Input: part model. Units: mm. Frame: model coordinates. A direction names the side the tool comes from. Round coordinates to 2 decimals unless told otherwise and drop trailing zeros. Loops run counter-clockwise (first coordinate to the right, second up) from the corner with the lowest first, then second, coordinate; pieces in that order, holes last. Notation, with made-up numbers: (-14.5, 50) - (5.5, 50) arc R18 ccw to (5.5, 59) - close; hole circle Ø2 at (-14.75, 70.5). An arc over 180 degrees is marked (long way). Write each question's results on one line, items separated by ' | '.
from build123d import *

# Parameters (mm, degrees)
SKETCH1_R               = 1.45
BOSS_EXTRUDE1_DEPTH     = 5
SKETCH2_R               = 1.45
BOSS_EXTRUDE2_DEPTH     = 2.6
SKETCH3_R               = 1.45
BOSS_EXTRUDE3_DEPTH     = 3
SKETCH5_W               = 3
SKETCH5_H               = 52.5
CHAMFER1_SIZE           = 1
SKETCH6_R               = 0.75
CUT_EXTRUDE1_DEPTH      = 5.0000001
CUT_EXTRUDE1_DEPTH_BACK = 5.0000001


with BuildPart() as part:
    # Sketch1 → Boss-Extrude1 (new body)
    with BuildSketch(Plane(origin=(0, 0, 0), x_dir=(0, 0, -1), z_dir=(1, 0, 0))):
        with BuildLine():
            Line((-4, 0), (-4, 6.5))
            ThreePointArc((-4, 6.5), (0, 10.5), (4, 6.5))
            Line((4, 6.5), (4, 0))
            ThreePointArc((4, 0), (0, -4), (-4, 0))
        make_face()
        with Locations((0, 6.5)):
            Circle(SKETCH1_R, mode=Mode.SUBTRACT)
    extrude(amount=BOSS_EXTRUDE1_DEPTH)

    # Sketch2 → Boss-Extrude2 (add)
    with BuildSketch(Plane(origin=(5, 0, 0), x_dir=(0, 0, -1), z_dir=(1, 0, 0))):
        with Locations((0, 0.05)):
            Circle(SKETCH2_R)
    extrude(amount=BOSS_EXTRUDE2_DEPTH)

    # Sketch3 → Boss-Extrude3 (add)
    with BuildSketch(Plane.ZY):
        with BuildLine():
            ThreePointArc((-4, 6.5), (0, 2.5), (4, 6.5))
            ThreePointArc((4, 6.5), (0, 10.5), (-4, 6.5))
        make_face()
        with Locations((0, 6.5)):
            Circle(SKETCH3_R, mode=Mode.SUBTRACT)
    extrude(amount=BOSS_EXTRUDE3_DEPTH)

    # Sketch5 → Revolve2 (revolve)
    with BuildSketch(Plane.XY):
        with Locations((2.5, 34.25)):
            Rectangle(SKETCH5_W, SKETCH5_H)
    revolve(axis=Axis((1, 60.5, 0), (0, -1, 0)))

    # Chamfer1
    chamfer1_edges = [part.edges().sort_by_distance(p)[0] for p in [
        (-2, 60.5, 0),
    ]]
    chamfer(chamfer1_edges, length=CHAMFER1_SIZE)

    # Sketch6 → Cut-Extrude1 (cut, two sides)
    with BuildSketch(Plane.XY) as cut_extrude1_sk:
        with Locations((1, 56.5)):
            Circle(SKETCH6_R)
        with Locations((1, 51.5)):
            Circle(SKETCH6_R)
        with Locations((1, 46.5)):
            Circle(SKETCH6_R)
        with Locations((1, 41.5)):
            Circle(SKETCH6_R)
        with Locations((1, 36.5)):
            Circle(SKETCH6_R)
    extrude(amount=CUT_EXTRUDE1_DEPTH, mode=Mode.SUBTRACT)
    extrude(cut_extrude1_sk.sketch, amount=-CUT_EXTRUDE1_DEPTH_BACK, mode=Mode.SUBTRACT)


solid = part.part
1. Line query: line 1 (Y direction, x = 1, z = -1.95); line 2 (X direction, y = 4, z = -1.5); line 3 (Y direction, x = 2.25, z = -1). Output: solid intervals per line, ascending. Write a range as [from, to].
Answer:
line 1: [-3.49, 35.75], [37.25, 40.75], [42.25, 45.75], [47.25, 50.75], [52.25, 55.75], [57.25, 60.5] | line 2: [-3, 5] | line 3: [-3.87, 5.45], [7.55, 60.5]
2. Section query C-C, the plane y = 36.5. Output: boundary loops of the cut face in (x, z).
Answer:
outline: (0.25, -2.9) - (0.25, 2.9) arc R3 ccw to start; (1.75, -2.9) arc R3 ccw to (1.75, 2.9) - close
3. Section query B-B, the plane y = 16. Output: boundary loops of the cut face in (x, z).
Answer:
outline: circle Ø6 at (1, 0)
4. Contact query for flat-ended pins moving along their axis: pin 1 (2 mm diameter, centred on x = 4.5, z = 0, fed in from +Y); pin 2 (2.5 mm diameter, centred on x = 1, y = 41.5, fed in from -Z); pin 3 (6 mm diameter, centred on x = 2, y = 46, fed in from +Z). Output: stop coordinate, or through.
Answer:
pin 1: y = 60 | pin 2: z = -3 | pin 3: z = 3
5. Section query A-A, the plane x = 1. Count the separate pieces of the cut face and the enclosed holes in it, plus the area to 3 significant figures.
Answer:
separate pieces: 6 | enclosed holes: 1 | area: 352 mm^2
6. Set-up query: faces 1 (the cylindrical face through (6.282, -1.366, 0.314)), 2 (the cylindrical face through (2, -4, 0)), 3 (the flat face through (-3, 4.8, -0.1)), 4 (the cylindrical face through (2.384, 34.675, -2.662)), 5 (the cylindrical face through (-0.72, 9.2, -2.95)). Return all of +Z, -Z, +X, -X, +Y, -Y with unobstructed straight access to the full face (end or side cutting, diameter ignored); none if empty.
Answer:
face 1: +X | face 2: +X, -X, -Y | face 3: +Z, -Z, -X, +Y, -Y | face 4: +Y | face 5: none
